```python
from build123d import *

# Parameters (mm, degrees)
SKETCH1_W           = 109
SKETCH1_H           = 60
BOSS_EXTRUDE1_DEPTH = 50
CUT_EXTRUDE1_DEPTH  = 500
SHELL2_T            = -2
CUT_EXTRUDE2_DEPTH  = 500
FILLET1_R           = 1
FILLET2_R           = 10
SKETCH4_R           = 28.5
CUT_EXTRUDE3_DEPTH  = 5


with BuildPart() as part:
    # Sketch1 → Boss-Extrude1 (new body)
    with BuildSketch(Plane(origin=(0, 0, 0), x_dir=(1, 0, 0), z_dir=(0, 1, 0))):
        with BuildLine():
            ThreePointArc((-348.004117683, 21.026446367), (-325.093541396, 91.023149879), (-266.754117683, 135.978067844))
            Line((-266.754117683, 135.978067844), (-348.004117683, 135.978067844))
            Line((-348.004117683, 135.978067844), (-348.004117683, 21.026446367))
        make_face()
        with BuildLine():
            Line((-266.754117683, -98.261932156), (-266.754117683, 135.978067844))
            ThreePointArc((-266.754117683, 135.978067844), (-325.093541396, 91.023149879), (-348.004117683, 21.026446367))
            Line((-348.004117683, 21.026446367), (-348.004117683, 16.688022305))
            ThreePointArc((-348.004117683, 16.688022305), (-325.094915866, -53.306736582), (-266.758579073, -98.261932156))
            Line((-266.758579073, -98.261932156), (-266.754117683, -98.261932156))
        make_face()
        with BuildLine():
            Line((-348.004117683, -98.261932156), (-266.758579073, -98.261932156))
            ThreePointArc((-266.758579073, -98.261932156), (-325.094915866, -53.306736582), (-348.004117683, 16.688022305))
            Line((-348.004117683, 16.688022305), (-348.004117683, -98.261932156))
        make_face()
        with BuildLine():
            Line((-266.743984385, 48.857234336), (-207.123984385, 48.857234336))
            Line((-207.123984385, 48.857234336), (-207.123984385, 142.874902464))
            ThreePointArc((-207.123984385, 142.874902464), (-237.359097186, 143.058210347), (-266.754117683, 135.978067844))
            Line((-266.754117683, 135.978067844), (-266.754117683, -98.261932156))
            Line((-266.754117683, -98.261932156), (-266.758579073, -98.261932156))
            ThreePointArc((-266.758579073, -98.261932156), (-237.361462745, -105.343468051), (-207.123984385, -105.160433792))
            Line((-207.123984385, -105.160433792), (-207.123984385, -11.142765664))
            Line((-207.123984385, -11.142765664), (-266.743984385, -11.142765664))
            Line((-266.743984385, -11.142765664), (-266.743984385, 48.857234336))
        make_face()
        with Locations((-212.243984385, 18.857234336)):
            Rectangle(SKETCH1_W, SKETCH1_H)
    extrude(amount=BOSS_EXTRUDE1_DEPTH)

    # Sketch2 → Cut-Extrude1 (cut)
    with BuildSketch(Plane.XY.offset(98.261932156)):
        Polygon((-348.004117683, 50), (-348.004117683, 10), (-323.004117683, 50), align=None)
        Polygon((-308.004117683, 25), (-333.004117683, 0), (-308.004117683, 0), align=None)
    extrude(amount=-CUT_EXTRUDE1_DEPTH, mode=Mode.SUBTRACT)

    # Shell2
    shell2_openings = [part.faces().sort_by_distance(p)[0] for p in [
        (-340.504117683, 0, -18.858067844),
    ]]
    offset(amount=SHELL2_T, openings=shell2_openings, kind=Kind.INTERSECTION)

    # Sketch3 → Cut-Extrude2 (cut)
    with BuildSketch(Plane.XY.offset(98.261932156)):
        Polygon((-348.004117683, 0), (-348.004117683, 4), (-340.004117683, 0), align=None)
    extrude(amount=-CUT_EXTRUDE2_DEPTH, mode=Mode.SUBTRACT)

    # Fillet1
    fillet1_edges = [part.edges().sort_by_distance(p)[0] for p in [
        (-348.004117683, 4, -18.858067844),
        (-346.004117683, 3, -18.858067844),
    ]]
    fillet(fillet1_edges, radius=FILLET1_R - 0.0001)  # a hair under: the kernel refuses the full size

    # Fillet2
    fillet2_edges = [part.edges().sort_by_distance(p)[0] for p in [
        (-340.004117683, 0, -134.978067844),
        (-340.004117683, 0, 97.261932156),
    ]]
    fillet(fillet2_edges, radius=FILLET2_R)

    # Sketch4 → Cut-Extrude3 (cut)
    with BuildSketch(Plane(origin=(0, 50, 0), x_dir=(1, 0, 0), z_dir=(0, 1, 0))):
        with Locations(Location((-237.743984385, 18.857234336, 0), (0, 0, 270))):
            Circle(SKETCH4_R)
    extrude(amount=-CUT_EXTRUDE3_DEPTH, mode=Mode.SUBTRACT)


solid = part.part
```
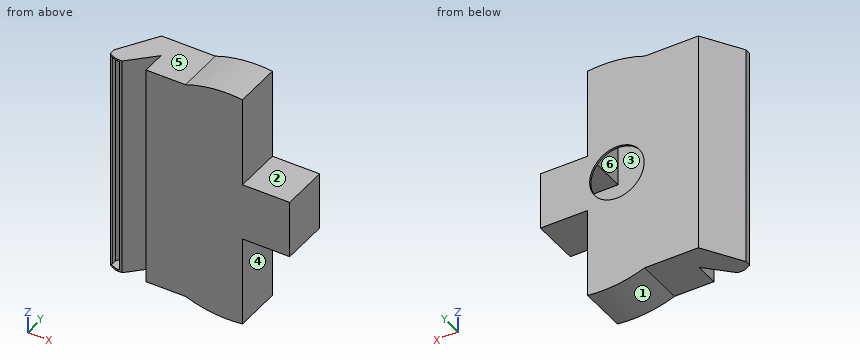
Could you check a few things on this model? Use its own coordinates, in mm. Face numbers are marked on the shaded views. A direction names the side the tool comes from. Round coordinates to 2 decimals unless told otherwise and drop trailing zeros. Write each loop counter-clockwise with the first axis right and the second up, starting at its lowest first coordinate (ties: lowest second). Pieces come first, ordered by that corner, then holes. Notation, with made-up numbers: M 55,-16 L 95,-16 A16 cw 95,15 Z; hole C 36,10 d11. An arc over 180 degrees is marked long. Write each question's results on one line, items separated by ' | '. Start each with the question number.
1. Imagine slicing it at A-A on y = 22. List the corners of the cut face in (x, z) for me, and give its area (3 significant figures).
2. Imagine slicing it at B-B on x = -274. List the corners of the cut face in (y, z) for me, and give its area (3 significant figures).
3. I'm going to push flat-ended pins straight in: pin 1 Ø14 at (y, z) = (27.5, 60) entering from -X; pin 2 Ø25 at (x, y) = (-318.5, 13.5) entering from +Z; pin 3 Ø10 at (x, y) = (-270.5, 6.5) entering from -Z. Where does each tip first touch, or does it pass through?
4. Imagine slicing it at D-D on y = 36. List the corners of the cut face in (x, z) for me, and give its area (3 significant figures).
5. I need wall thicknesses on L1, parallel to Z at x = -332, y = 16.5; L2, parallel to Z at x = -179, y = 31.5; L3, parallel to Y at x = -259, z = 67.5. Which ranges of each line are inside material? Lowest first, please. Write a range as from..to.
6. On a 3-axis mill with a long thin cutter (end or side, diameter ignored), from which of +Z, -Z, +X, -X, +Y, -Y can I reach the whole of each face in a straight line? I mean the marked faces 4, 5 and 6. Say none if no direction works.
7. Thinking about a two-plate mould opening in Z: for the marked faces 1, 2 and 3, which applies, +Z half, -Z half, draft (parallel to the pull), parting line (faces both ways), or undercut?
Result sheet:
1) outline: M -340.5,-135.98 L -311,-135.98 L -311,98.26 L -340.5,98.26 Z; M -308,-135.98 L -266.75,-135.98 A125.03 ccw -207.12,-142.87 L -207.12,-48.86 L -157.74,-48.86 L -157.74,11.14 L -207.12,11.14 L -207.12,105.16 A125.03 ccw -266.76,98.26 L -308,98.26 Z; hole M -338.15,-133.98 L -313.83,-133.98 L -313.83,96.26 L -338.15,96.26 Z; hole M -306,-133.98 L -266.39,-133.98 A123.03 ccw -209.12,-141.1 L -209.12,-46.86 L -159.74,-46.86 L -159.74,9.14 L -209.12,9.14 L -209.12,103.39 A123.03 ccw -266.4,96.26 L -306,96.26 Z | area: 2,870 mm^2
2) outline: M 0,-135.98 L 50,-135.98 L 50,98.26 L 0,98.26 Z; hole M 2,-133.98 L 48,-133.98 L 48,96.26 L 2,96.26 Z | area: 1,120 mm^2
3) pin 1: stops at x = -341.44 | pin 2: stops at z = 98.26 | pin 3: stops at z = -136.44
4) outline: M -331.75,-135.98 L -266.75,-135.98 A125.03 ccw -207.12,-142.87 L -207.12,-48.86 L -157.74,-48.86 L -157.74,11.14 L -207.12,11.14 L -207.12,105.16 A125.03 ccw -266.76,98.26 L -331.75,98.26 Z; hole M -329.4,-133.98 L -266.39,-133.98 A123.03 ccw -209.12,-141.1 L -209.12,-46.86 L -159.74,-46.86 L -159.74,9.14 L -209.12,9.14 L -209.12,103.39 A123.03 ccw -266.4,96.26 L -329.4,96.26 Z | area: 1,730 mm^2
5) L1: z = -135.98..-133.98, 96.26..98.26 | L2: z = -48.86..-46.86, 9.14..11.14 | L3: y = 0..2, 48..50
6) face 4: -Z, +X, +Y, -Y | face 5: +Z, -X, +Y, -Y | face 6: none
7) face 1: -Z half | face 2: +Z half | face 3: undercut
